Could you check a few things on this model? Use its own coordinates, in mm. Face numbers are marked on the shaded views. A direction names the side the tool comes from. Coordinates: 2 decimals unless noted, no trailing zeros. One line per item, written item: value. Start each with the question number.
(1) On a 3-axis mill with a long thin cutter (end or side, diameter ignored), from which of +Z, -Z, +X, -X, +Y, -Y can I reach the whole of each face in a straight line? I mean the marked faces 1, 2 and 3. Say none if no direction works.
(2) If I drill on line 1 along X through (y, z) = (54, 22); line 2 along X through (y, z) = (31, -2.5), over which ranges is the centre line in solid material (lowest first)? Write a range as from..to.
(3) I'm going to push flat-ended pins straight in: P1, Ø4, axis at y = 51, z = 3, coming from the +X side; P2, Ø10, axis at y = 28.5, z = -6, coming from the +X side; P3, Ø8, axis at x = -24.5, z = -21, coming from the -Y side. Where does each tip first touch, or does it pass through?
(4) If we mould it in two halves opening along X, with no side actions, what happens to the marked faces 4, 5 and 6? For each: pulls with the +X half, pulls with the -X half, needs draft (parallel to the pull), parting line crosses it, or undercut.
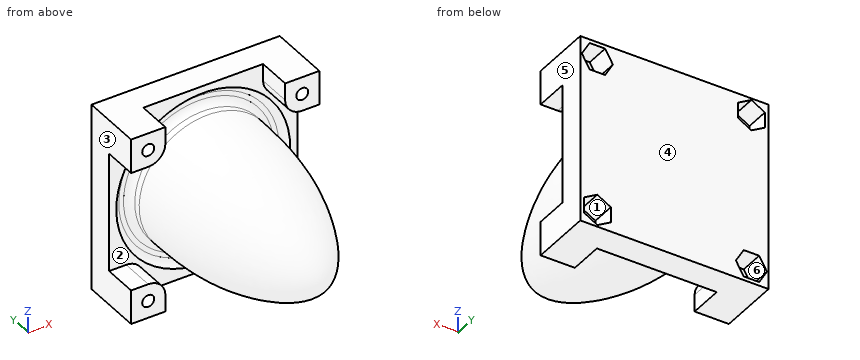
```python
from build123d import *

# Parameters (mm, degrees)
SKETCH5_W           = 55
SKETCH5_H           = 70
BOSS_EXTRUDE8_DEPTH = 27.5
SKETCH6_W           = 10
SKETCH6_H           = 10
BOSS_EXTRUDE9_DEPTH = 10
SKETCH7_R           = 1.75
CUT_EXTRUDE2_DEPTH  = 59.723930461
CUT_EXTRUDE3_DEPTH  = 7
CIRPATTERN1_COUNT   = 4
FILLET1_R           = 5


with BuildPart() as part:
    # Sketch5 → Boss-Extrude8 (new, symmetric)
    with BuildSketch(Plane.XY):
        with Locations((0, 30)):
            Rectangle(SKETCH5_W, SKETCH5_H)
    extrude(amount=BOSS_EXTRUDE8_DEPTH, both=True)

    # Sketch1 → Cut-Revolve1 (revolve, cut)
    with BuildSketch(Plane(origin=(0, 0, 0), x_dir=(0, 0, -1), z_dir=(1, 0, 0))):
        with BuildLine():
            Line((0, -7), (0, 3))
            add(Edge.make_bspline(
                [(20, 55), (20, 43.957678864), (18.5157836, 25.942674232), (6.738040747, 3), (0, 3)],
                knots=[0, 0, 0, 0, 0.518417095, 1, 1, 1, 1], degree=3))
            Line((20, 55), (20, 57))
            ThreePointArc((20, 57), (20.585786438, 58.414213562), (22, 59))
            Line((22, 59), (23.4, 59))
            ThreePointArc((23.4, 59), (24.814213562, 58.414213562), (25.4, 57))
            Line((25.4, 57), (304.80691679, 57))
            Line((304.80691679, 57), (304.80691679, -311.267440696))
            Line((304.80691679, -311.267440696), (0, -311.267440696))
            Line((0, -311.267440696), (0, -7))
        make_face()
    revolve(axis=Axis((0, 0, 0), (0, 1, 0)), mode=Mode.SUBTRACT)

    # Sketch6 → Boss-Extrude9 (add)
    with BuildSketch(Plane.XZ.offset(-57)):
        with Locations((-22.5, 22.5)):
            Rectangle(SKETCH6_W, SKETCH6_H)
    boss_extrude9 = extrude(amount=BOSS_EXTRUDE9_DEPTH)

    # Sketch7 → Cut-Extrude2 (cut, through all)
    with BuildSketch(Plane.XZ.offset(-47)):
        with Locations(Location((-22.5, 22.5, 0), (0, 0, 270))):
            Circle(SKETCH7_R)
    cut_extrude2 = extrude(amount=-CUT_EXTRUDE2_DEPTH, mode=Mode.SUBTRACT)

    # Sketch8 → Cut-Extrude3 (cut)
    with BuildSketch(Plane(origin=(0, 65, 0), x_dir=(1, 0, 0), z_dir=(0, 1, 0))):
        Polygon((-22.5, -17.962026884), (-26.43, -20.231013442), (-26.43, -24.768986558), (-22.5, -27.037973116), (-18.57, -24.768986558), (-18.57, -20.231013442), align=None)
    cut_extrude3 = extrude(amount=-CUT_EXTRUDE3_DEPTH, mode=Mode.SUBTRACT)

    # CirPattern1: Boss-Extrude9, Cut-Extrude2, Cut-Extrude3 ×4 about axis
    cirpattern1_axis = Axis((0, 0, 0), (0, 1, 0))
    add([boss_extrude9.rotate(cirpattern1_axis, i * 360 / CIRPATTERN1_COUNT) for i in range(1, CIRPATTERN1_COUNT)])
    add([cut_extrude2.rotate(cirpattern1_axis, i * 360 / CIRPATTERN1_COUNT) for i in range(1, CIRPATTERN1_COUNT)], mode=Mode.SUBTRACT)
    add([cut_extrude3.rotate(cirpattern1_axis, i * 360 / CIRPATTERN1_COUNT) for i in range(1, CIRPATTERN1_COUNT)], mode=Mode.SUBTRACT)

    # Fillet1
    # the kernel refuses this fillet: 5 mm, written as the material it takes off along each edge
    with BuildSketch(Plane(origin=(-17.5, 57, 17.5), x_dir=(0, 0, 1), z_dir=(0, -1, 0)), Plane(origin=(17.5, 57, 17.5), x_dir=(1, 0, 0), z_dir=(0, -1, 0))) as fillet1_piece_1:
        with BuildLine():
            CenterArc((FILLET1_R, FILLET1_R), FILLET1_R, 180, 90)
            Line((0, FILLET1_R), (0, 0))
            Line((0, 0), (FILLET1_R, 0))
        make_face()
    extrude(amount=22.5, mode=Mode.SUBTRACT)
    with BuildSketch(Plane(origin=(-17.5, 57, -17.5), x_dir=(0, 0, -1), z_dir=(0, -1, 0)), Plane(origin=(17.5, 57, -17.5), x_dir=(1, 0, 0), z_dir=(0, -1, 0))) as fillet1_piece_2:
        with BuildLine():
            CenterArc((FILLET1_R, -FILLET1_R), FILLET1_R, 90, 90)
            Line((0, -FILLET1_R), (0, 0))
            Line((0, 0), (FILLET1_R, 0))
        make_face()
    extrude(amount=22.5, mode=Mode.SUBTRACT)


solid = part.part
```
Values:
1. face 1: +Y
1. face 2: -Y
1. face 3: +Z, -Z, -X, +Y, -Y
2. line 1: x = -27.5..-24.18, -20.82..-17.53, 17.53..20.82, 24.18..27.5
2. line 2: x = -17.51..17.51
3. P1: stops at x = 19.94
3. P2: stops at x = 17.77
3. P3: stops at y = 47
4. face 4: needs draft
4. face 5: pulls with the +X half
4. face 6: undercut
